The drawing under review shows one solid part. Ordinate dimensions are in mm from its lowest x, y, z. Coordinates: 2 decimals unless noted, no trailing zeros. Write each loop counter-clockwise with the first axis right and the second up, starting at its lowest first coordinate (ties: lowest second). Pieces come first, ordered by that corner, then holes.
Q1. Insertion check: pin 1 (5 mm diameter, centred on y = 20, z = 65, fed in from -X); pin 2 (1.7 mm diameter, centred on x = 2, z = 68, fed in from -Y); pin 3 (1.9 mm diameter, centred on y = 20, z = 5, fed in from -X); pin 4 (2.5 mm diameter, centred on x = 3.5, y = 11.5, fed in from +Z). Each pin has a flat end and moves straight along its axis. Give the tip position at first contact, or say it passes through.
Q2. For probe 1 along Y at (x, z) = (3.45, 49); probe 2 along Z at (x, y) = (4.45, 16); probe 3 along Y at (x, z) = (2.3, 9.5), list the stretches that pass through material, from the lowest coordinate up.
Q3. Take a section at B-B (y = 64.5). Give the boundary of the cut face in (x, z).
Q4. Take a section at C-C (z = 15.5). Give the boundary of the cut face in (x, y).
Q5. Take a section at A-A (x = 3.8). Give the boundary of the cut face in (y, z) (1 decimal), and give its area (3 significant figures).
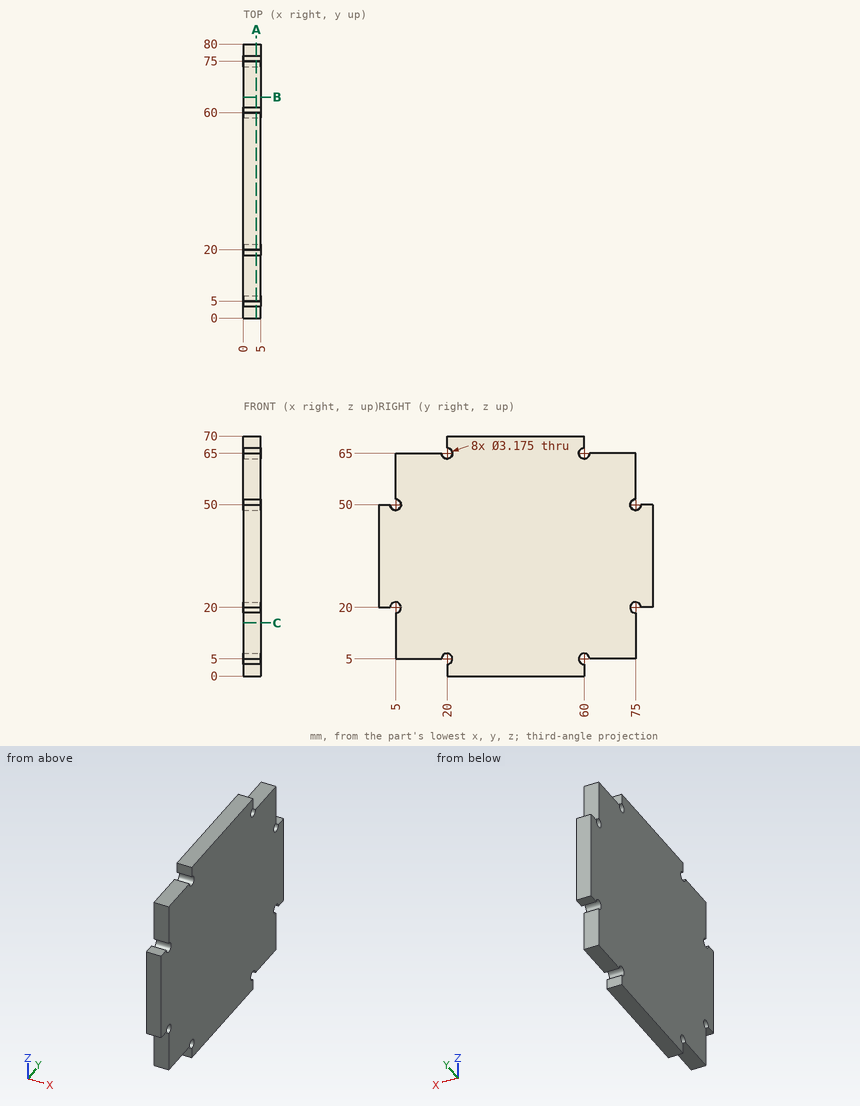
Response:
1. pin 1: stops at x = 0
1. pin 2: stops at y = 20
1. pin 3: passes through
1. pin 4: stops at z = 65
2. probe 1: y = 0 to 3.77, 6.23 to 73.77, 76.23 to 80
2. probe 2: z = 5 to 65
2. probe 3: y = 5 to 75
3. outline: (0, 5) - (5, 5) - (5, 65) - (0, 65) - close
4. outline: (0, 5) - (5, 5) - (5, 75) - (0, 75) - close
5. outline: (0, 20) - (3.4, 20) arc R1.6 cw (long way) to (5, 18.4) - (5, 5) - (18.4, 5) arc R1.6 cw (long way) to (20, 3.4) - (20, 0) - (60, 0) - (60, 3.4) arc R1.6 cw (long way) to (61.6, 5) - (75, 5) - (75, 18.4) arc R1.6 cw (long way) to (76.6, 20) - (80, 20) - (80, 50) - (76.6, 50) arc R1.6 cw (long way) to (75, 51.6) - (75, 65) - (61.6, 65) arc R1.6 cw (long way) to (60, 66.6) - (60, 70) - (20, 70) - (20, 66.6) arc R1.6 cw (long way) to (18.4, 65) - (5, 65) - (5, 51.6) arc R1.6 cw (long way) to (3.4, 50) - (0, 50) - close
5. area: 4,850 mm2
